Could you check a few things on this model? Use its own coordinates, in mm. Face numbers are marked on the shaded views. Round coordinates to 2 decimals unless told otherwise and drop trailing zeros. Loops run counter-clockwise (first coordinate to the right, second up) from the corner with the lowest first, then second, coordinate; pieces in that order, holes last. Notation, with made-up numbers: (20.5, -36.5) -> (75.5, -36.5) arc R8 cw to (75.5, -22.5) -> close; hole circle Ø8 at (-27, 2.5). An arc over 180 degrees is marked (long way). One line per item, written item: value.
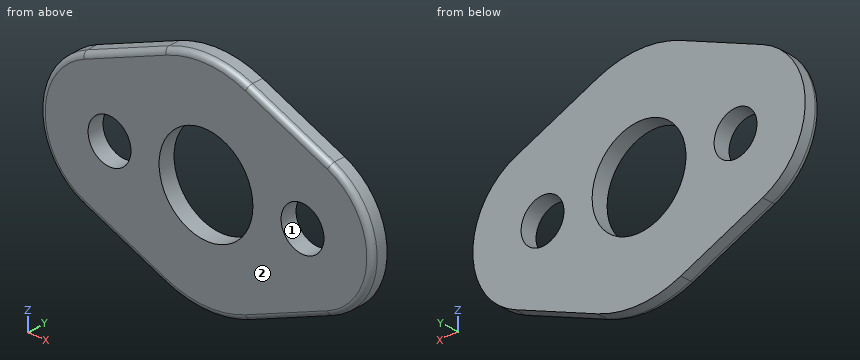
```python
from build123d import *

# Parameters (mm, degrees)
F0_R     = 4
F0_R_2   = 8.75
F1_DEPTH = 3
F2_R     = 1


with BuildPart() as f1:
    # F0 (on Front) → F1 (new body)
    with BuildSketch(Plane.XZ):
        with BuildLine():
            Line((-23.055556, -11.976701), (-7.777778, -18.425693))
            ThreePointArc((-7.777778, -18.425693), (0, -20), (7.777778, -18.425693))
            Line((7.777778, -18.425693), (23.055556, -11.976701))
            ThreePointArc((23.055556, -11.976701), (31, 0), (23.055556, 11.976701))
            Line((23.055556, 11.976701), (7.777778, 18.425693))
            ThreePointArc((7.777778, 18.425693), (0, 20), (-7.777778, 18.425693))
            Line((-7.777778, 18.425693), (-23.055556, 11.976701))
            ThreePointArc((-23.055556, 11.976701), (-31, 0), (-23.055556, -11.976701))
        make_face()
        with Locations((-18, 0)):
            Circle(F0_R, mode=Mode.SUBTRACT)
        Circle(F0_R_2, mode=Mode.SUBTRACT)
        with Locations((18, 0)):
            Circle(F0_R, mode=Mode.SUBTRACT)
    extrude(amount=F1_DEPTH)

    # F2
    f2_edges = [f1.edges().sort_by_distance(p)[0] for p in [
        (15.416667, -3, 15.201197),
    ]]
    fillet(f2_edges, radius=F2_R)


solid = f1.part
```
Item 1: If we section it at A-A on z = 0: List the corners of the cut face in (x, y) for me, plus the area to 3 significant figures.
Output:
outline: (-31, -2) arc R1 ccw to (-30, -3) -> (-22, -3) -> (-22, 0) -> (-31, 0) -> close; (-14, -3) -> (-8.75, -3) -> (-8.75, 0) -> (-14, 0) -> close; (8.75, -3) -> (14, -3) -> (14, 0) -> (8.75, 0) -> close; (22, -3) -> (30, -3) arc R1 ccw to (31, -2) -> (31, 0) -> (22, 0) -> close
area: 85.1 mm²
Item 2: If we mould it in two halves opening along Z, with no side actions, what happens to the marked faces 1 and 2? For each: released by +Z, released by -Z, zero draft, split by the parting line, or undercut.
Output:
face 1: undercut
face 2: zero draft
Item 3: If we section it at C-C on x = 0: List the corners of the cut face in (y, z) for me.
Output:
outline: (-3, -19) arc R1 ccw to (-2, -20) -> (0, -20) -> (0, -8.75) -> (-3, -8.75) -> close; (-3, 8.75) -> (0, 8.75) -> (0, 20) -> (-2, 20) arc R1 ccw to (-3, 19) -> close
Item 4: Will these pins go through, and if not, where does the flat tip stop? pin 1 Ø1.5 at (y, z) = (-1, 8.5) entering from -X; pin 2 Ø1 at (y, z) = (-1, 14) entering from +X.
Output:
pin 1: stops at x = -28.44
pin 2: stops at x = 19.45
Item 5: If we section it at B-B on y = -1: List the corners of the cut face in (x, z) for me.
Output:
outline: (-23.06, -11.98) -> (-7.78, -18.43) arc R20 ccw to (7.78, -18.43) -> (23.06, -11.98) arc R13 ccw to (23.06, 11.98) -> (7.78, 18.43) arc R20 ccw to (-7.78, 18.43) -> (-23.06, 11.98) arc R13 ccw to start; hole circle Ø8 at (-18, 0); hole circle Ø17.5 at (0, 0); hole circle Ø8 at (18, 0)
Item 6: I need wall thicknesses on line 1 (X direction, y = -2.3, z = -0.5); line 2 (Z direction, x = -18, y = -0.9); line 3 (Z direction, x = 4, y = -0.6). Which ranges of each line are inside material? Lowest first, please. Write a range as from..to.
Output:
line 1: x = -30.94..-21.97, -14.03..-8.74, 8.74..14.03, 21.97..30.94
line 2: z = -14.11..-4, 4..14.11
line 3: z = -19.6..-7.78, 7.78..19.6
